from build123d import *

# Parameters (mm, degrees)
BOSS_EXTRUDE1_DEPTH = 6
CUT_EXTRUDE1_DEPTH  = 6
CUT_EXTRUDE3_DEPTH  = 2
FILLET1_R           = 3


with BuildPart() as part:
    # Sketch1 → Boss-Extrude1 (new body)
    with BuildSketch(Plane.XY):
        Polygon((10, 0), (45.087262032, 0.612450437), (45, 5.611688913), (9.912737968, 4.999238476), (0.087262032, 4.999238476), (-35, 5.611688913), (-35.087262032, 0.612450437), (0, 0), (0, -2), (10, -2), align=None)
    extrude(amount=BOSS_EXTRUDE1_DEPTH)

    # Sketch2 → Cut-Extrude1 (cut)
    with BuildSketch(Plane(origin=(0.087262032, 4.999238476, 0), x_dir=(0.9998476951563913, -0.017452406437283737, 0), z_dir=(0.017452406437283737, 0.9998476951563913, 0))):
        with BuildLine():
            Line((-29.092606806, -4.2), (-24.692606806, -4.2))
            ThreePointArc((-24.692606806, -4.2), (-23.492606806, -3), (-24.692606806, -1.8))
            Line((-24.692606806, -1.8), (-29.092606806, -1.8))
            ThreePointArc((-29.092606806, -1.8), (-30.292606806, -3), (-29.092606806, -4.2))
        make_face()
    cut_extrude1 = extrude(amount=-CUT_EXTRUDE1_DEPTH, mode=Mode.SUBTRACT)

    # Sketch2<3> → Cut-Extrude3 (cut)
    with BuildSketch(Plane(origin=(0.087262032, 4.999238476, 0), x_dir=(0.9998476951563913, -0.017452406437283737, 0), z_dir=(0.017452406437283737, 0.9998476951563913, 0))):
        Polygon((-22.492606806, -3), (-23.592606806, -1.094744112), (-30.192606806, -1.094744112), (-31.292606806, -3), (-30.192606806, -4.905255888), (-23.592606806, -4.905255888), align=None)
        with BuildLine():
            ThreePointArc((-24.692606806, -4.2), (-23.492606806, -3), (-24.692606806, -1.8))
            Line((-24.692606806, -1.8), (-29.092606806, -1.8))
            ThreePointArc((-29.092606806, -1.8), (-30.292606806, -3), (-29.092606806, -4.2))
            Line((-29.092606806, -4.2), (-24.692606806, -4.2))
        make_face(mode=Mode.SUBTRACT)
    cut_extrude3 = extrude(amount=-CUT_EXTRUDE3_DEPTH, mode=Mode.SUBTRACT)

    # Mirror1: Cut-Extrude1, Cut-Extrude3 across plane
    add(cut_extrude1.mirror(Plane(origin=(5, 0, 0), x_dir=(0, 0, 1), z_dir=(1, 0, 0))), mode=Mode.SUBTRACT)
    add(cut_extrude3.mirror(Plane(origin=(5, 0, 0), x_dir=(0, 0, 1), z_dir=(1, 0, 0))), mode=Mode.SUBTRACT)

    # Fillet1
    fillet1_edges = [part.edges().sort_by_distance(p)[0] for p in [
        (45.043631016, 3.112069675, 0),
        (45.043631016, 3.112069675, 6),
        (-35.043631016, 3.112069675, 0),
        (-35.043631016, 3.112069675, 6),
    ]]
    fillet(fillet1_edges, radius=FILLET1_R - 0.0001)  # a hair under: the kernel refuses the full size


solid = part.part
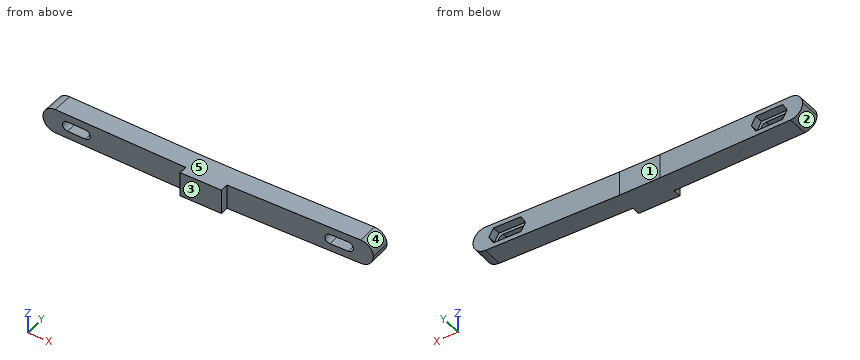
For this review, take the finished solid that the model builds, in its own axes (mm). Face numbers are marked on the shaded views. A direction names the side the tool comes from. Round coordinates to 2 decimals unless told otherwise and drop trailing zeros. Loops run counter-clockwise (first coordinate to the right, second up) from the corner with the lowest first, then second, coordinate; pieces in that order, holes last. Notation, with made-up numbers: (20.25, 11.25) - (76.25, 11.25) arc R23 ccw to (76.25, 37.25) - close; hole circle Ø1 at (41.5, -34.5). An arc over 180 degrees is marked (long way). One line per question, with ' | ' between items.
Q1. The part is to be moulded in two halves that separate along X. For the marked faces 1, 2 and 3, say which applies: released by +X, released by -X, zero draft, split by the parting line, or undercut.
Taken from the geometry:
face 1: undercut | face 2: released by -X | face 3: zero draft
Q2. For pin 1 (3 mm diameter, centred on x = -7, z = 1.5, fed in from +Y); pin 2 (0.6 mm diameter, centred on y = -1, z = 2, fed in from -X); pin 3 (0.6 mm diameter, centred on y = -0.5, z = 3, fed in from +X), all flat-tipped, find the tip position at first contact; note any pin that passes through.
Taken from the geometry:
pin 1: stops at y = 5.15 | pin 2: stops at x = 0 | pin 3: stops at x = 10
Q3. Take a section at A-A (x = -27.5). Give the boundary of the cut face in (y, z), and give its area (3 significant figures).
Taken from the geometry:
outline: (0.48, 0) - (5.48, 0) - (5.48, 1.09) - (3.48, 1.09) - (3.48, 1.8) - (0.48, 1.8) - close; (0.48, 4.2) - (3.48, 4.2) - (3.48, 4.91) - (5.48, 4.91) - (5.48, 6) - (0.48, 6) - close | area: 15.2 mm²
Q4. Tool access review of the marked faces 4 and 5: name each direction out of +Z, -Z, +X, -X, +Y, -Y from which nothing blocks a thin tool from reaching the whole face with its end or side.
Taken from the geometry:
face 4: +Z, +X, +Y | face 5: +Z, +X, -X, +Y, -Y
Q5. Take a section at B-B (x = 21.5). Give the boundary of the cut face in (y, z), and give its area (3 significant figures).
Taken from the geometry:
outline: (0.2, 0) - (5.2, 0) - (5.2, 6) - (0.2, 6) - close | area: 30.0 mm²
Q6. For line 1 along X through (y, z) = (3.25, 2); line 2 along Z through (x, y) = (35, 5); line 3 along Z through (x, y) = (-26, 1), list the stretches that pass through material, from the lowest coordinate up. Write a range as [from, to].
Taken from the geometry:
line 1: x = [-34.87, -29.7], [-23.98, 33.98], [39.7, 44.87] | line 2: z = [0, 1.09], [4.91, 6] | line 3: z = [0, 1.8], [4.2, 6]
